```python
from build123d import *

# Parameters (mm, degrees)
F2_DEPTH = 5
F4_DEPTH = 4
F6_DEPTH = 5


with BuildPart() as f2:
    # F1 (on Top) → F2 (new body)
    with BuildSketch(Plane.XY):
        Polygon((-20.4275340124, 94.3563715087), (-20.4275340124, 89.3563715087), (-15.4275340124, 89.3563715087), (-4.7150340124, 89.3563715087), (2.3560337995, 89.3563715087), (10.9974659876, 89.3563715087), (10.9974659876, 94.3563715087), align=None)
        Polygon((-15.4275340124, 89.3563715087), (-20.4275340124, 89.3563715087), (-20.4275340124, 39.3563715087), (-15.4275340124, 39.3563715087), (-15.4275340124, 71.5728036968), (-15.4275340124, 78.6438715087), align=None)
        Polygon((-4.7150340124, 89.3563715087), (-15.4275340124, 78.6438715087), (-15.4275340124, 71.5728036968), (2.3560337995, 89.3563715087), align=None)
    extrude(amount=F2_DEPTH)

    # F3 (on face) → F4 (join)
    with BuildSketch(Plane(origin=(0, 94.3563715087, 0), x_dir=(-1, 0, 0), z_dir=(0, 1, 0))):
        with BuildLine():
            ThreePointArc((-8.3974659876, 2.5), (-9.6974659876, 3.8), (-10.9974659876, 2.5))
            Line((-10.9974659876, 2.5), (-8.3974659876, 2.5))
        make_face()
        with BuildLine():
            Line((-8.3974659876, 2.5), (-10.9974659876, 2.5))
            ThreePointArc((-10.9974659876, 2.5), (-9.6974659876, 1.2), (-8.3974659876, 2.5))
        make_face()
        with BuildLine():
            Line((20.4275340124, 2.5), (17.8275340124, 2.5))
            ThreePointArc((17.8275340124, 2.5), (19.1275340124, 1.2), (20.4275340124, 2.5))
        make_face()
        with BuildLine():
            ThreePointArc((20.4275340124, 2.5), (19.1275340124, 3.8), (17.8275340124, 2.5))
            Line((17.8275340124, 2.5), (20.4275340124, 2.5))
        make_face()
    extrude(amount=F4_DEPTH)

    # F5 (on face) → F6 (cut, through all)
    with BuildSketch(Plane(origin=(0, 0, 0), x_dir=(1, 0, 0), z_dir=(0, 0, -1))):
        Polygon((-15.4275340124, -39.3563715087), (-17.9275340124, -39.3563715087), (-15.4275340124, -48.7645578384), align=None)
        Polygon((-20.4275340124, -48.7645578384), (-17.9275340124, -39.3563715087), (-20.4275340124, -39.3563715087), align=None)
        Polygon((-19.0904904157, -47.5493085384), (-20.4275340124, -48.7645578384), (-20.4275340124, -56.3598138094), align=None)
        Polygon((-15.4275340124, -56.3598138094), (-15.4275340124, -48.7645578384), (-16.8119128793, -47.5493085384), align=None)
        Polygon((-15.4275340124, -64.1069722176), (-15.4275340124, -56.3598138094), (-16.8119128793, -55.2964669466), align=None)
        Polygon((-19.0904904157, -55.2964669466), (-20.4275340124, -56.3598138094), (-20.4275340124, -64.1069722176), align=None)
    extrude(amount=-F6_DEPTH, mode=Mode.SUBTRACT)


solid = f2.part
```
Work out the finished part from the listing and answer in its coordinate system (mm). A direction names the side the tool comes from. Coordinates: 2 decimals unless noted, no trailing zeros. Write each loop counter-clockwise with the first axis right and the second up, starting at its lowest first coordinate (ties: lowest second). Pieces come first, ordered by that corner, then holes.
Q1. Which of the six approach directions +Z, -Z, +X, -X, +Y, -Y give full straight-line access (tool end or side, diameter ignored) to faces 4 (the face through (-15.428, 68, 2)), 5 (the face through (-20.328, 96.328, 2.002)), 6 (the face through (-15.428, 84, 2))?
Q2. A cutting plane is placed at D-D, the plane y = 70. Give the vertices of the cut face in (x, z).
Q3. A cutting plane is placed at C-C, the plane x = -16. Give the vertices of the cut face in (y, z).
Q4. Find the intervals of material crossed by line 1 (Y direction, x = 3, z = 1.75); line 2 (Y direction, x = -6, z = 3.1); line 3 (X direction, y = 85.5, z = 4.5), in increasing order.
Q5. A cutting plane is placed at B-B, the plane x = -10. Give the vertices of the cut face in (y, z).
Q6. Each of these flat-tipped pins is pushed along its axis until it touches: pin 1 Ø3 at (x, z) = (-2.5, 3.5) entering from -Y; pin 2 Ø2.5 at (y, z) = (68.5, 3.5) entering from +X; pin 3 Ø1.5 at (x, z) = (-13, 3) entering from +Y; pin 4 Ø10 at (x, y) = (-10.5, 58.5) entering from +Z. Where does it stop, or does it pass through?
Q7. Determine the mould class of faces 1 (the face through (-10, 89.356, 2)), 2 (the face through (-12, 79, 0)), 3 (the face through (-7, 80, 2)) for opening direction X: released by +X, released by -X, zero draft, split by the parting line, or undercut.
Q8. A cutting plane is placed at A-A, the plane z = 0.6. Give the vertices of the cut face in (x, y), then the cut area to 3 significant figures.
Findings below:
1. face 4: +Z, -Z, +X, -Y
1. face 5: +Y
1. face 6: +Z, -Z
2. outline: (-20.43, 0) - (-15.43, 0) - (-15.43, 5) - (-20.43, 5) - close
3. outline: (46.61, 0) - (48.26, 0) - (48.26, 5) - (46.61, 5) - close; (52.72, 0) - (55.92, 0) - (55.92, 5) - (52.72, 5) - close; (60.46, 0) - (94.36, 0) - (94.36, 5) - (60.46, 5) - close
4. line 1: y = 89.36 to 94.36
4. line 2: y = 81 to 88.07, 89.36 to 94.36
4. line 3: x = -20.43 to -15.43, -8.57 to -1.5
5. outline: (77, 0) - (84.07, 0) - (84.07, 5) - (77, 5) - close; (89.36, 0) - (94.36, 0) - (94.36, 5) - (89.36, 5) - close
6. pin 1: stops at y = 83
6. pin 2: stops at x = -15.43
6. pin 3: stops at y = 94.36
6. pin 4: passes through
7. face 1: undercut
7. face 2: zero draft
7. face 3: released by +X
8. outline: (-20.43, 48.76) - (-17.93, 39.36) - (-15.43, 48.76) - (-16.81, 47.55) - (-15.43, 56.36) - (-16.81, 55.3) - (-15.43, 64.11) - (-15.43, 71.57) - (2.36, 89.36) - (11, 89.36) - (11, 94.36) - (-20.43, 94.36) - (-20.43, 64.11) - (-19.09, 55.3) - (-20.43, 56.36) - (-19.09, 47.55) - close; hole (-15.43, 78.64) - (-4.72, 89.36) - (-15.43, 89.36) - close
8. area: 463 mm2
